from build123d import *

# Parameters (mm, degrees)
SKETCH1_R           = 2.9845
SKETCH1_R_2         = 7.9375
SKETCH1_R_3         = 1.524
SKETCH1_R_4         = 7.250000001
BOSS_EXTRUDE1_DEPTH = 6.35
SKETCH1_3_R         = 7.9375
SKETCH1_3_R_2       = 7.250000001
CUT_EXTRUDE1_DEPTH  = 4.699


with BuildPart() as part:
    # Sketch1 → Boss-Extrude1 (new body)
    # profile 1 of 2: a face of its own
    with BuildSketch(Plane.XY):
        with BuildLine():
            Line((191.225613804, 305.383854225), (112.575613802, 305.383854225))
            ThreePointArc((112.575613802, 305.383854225), (110.330549772, 304.453918255), (109.400613802, 302.208854225))
            Line((109.400613802, 302.208854225), (109.400613802, 218.558854223))
            ThreePointArc((109.400613802, 218.558854223), (110.330549772, 216.313790192), (112.575613802, 215.383854223))
            Line((112.575613802, 215.383854223), (191.225613804, 215.383854223))
            ThreePointArc((191.225613804, 215.383854223), (193.470677834, 216.313790192), (194.400613804, 218.558854223))
            Line((194.400613804, 218.558854223), (194.400613804, 302.208854225))
            ThreePointArc((194.400613804, 302.208854225), (193.470677834, 304.453918255), (191.225613804, 305.383854225))
        make_face()
        with Locations((119.400613802, 245.383854222)):
            Circle(SKETCH1_R, mode=Mode.SUBTRACT)
        with Locations((149.400613802, 245.383854222)):
            Circle(SKETCH1_R, mode=Mode.SUBTRACT)
        with Locations((179.400613802, 225.383854222)):
            Circle(SKETCH1_R_2, mode=Mode.SUBTRACT)
        with Locations((168.605613802, 225.383854222)):
            Circle(SKETCH1_R_3, mode=Mode.SUBTRACT)
        with BuildLine():
            ThreePointArc((119.650613802, 265.633854223), (117.900613802, 263.883854223), (119.650613802, 262.133854222))
            Line((119.650613802, 262.133854222), (128.150613802, 262.133854222))
            ThreePointArc((128.150613802, 262.133854222), (129.900613803, 263.883854223), (128.150613802, 265.633854223))
            Line((128.150613802, 265.633854223), (119.650613802, 265.633854223))
        make_face(mode=Mode.SUBTRACT)
        with BuildLine():
            ThreePointArc((159.150613804, 262.133854222), (160.900613804, 263.883854223), (159.150613804, 265.633854223))
            Line((159.150613804, 265.633854223), (150.650613804, 265.633854223))
            ThreePointArc((150.650613804, 265.633854223), (148.900613803, 263.883854223), (150.650613804, 262.133854222))
            Line((150.650613804, 262.133854222), (159.150613804, 262.133854222))
        make_face(mode=Mode.SUBTRACT)
        with BuildLine():
            ThreePointArc((119.650613802, 296.633854224), (117.900613802, 294.883854224), (119.650613802, 293.133854224))
            Line((119.650613802, 293.133854224), (128.150613802, 293.133854224))
            ThreePointArc((128.150613802, 293.133854224), (129.900613803, 294.883854224), (128.150613802, 296.633854224))
            Line((128.150613802, 296.633854224), (119.650613802, 296.633854224))
        make_face(mode=Mode.SUBTRACT)
        with BuildLine():
            ThreePointArc((159.150613804, 293.133854224), (160.900613804, 294.883854224), (159.150613804, 296.633854224))
            Line((159.150613804, 296.633854224), (150.650613804, 296.633854224))
            ThreePointArc((150.650613804, 296.633854224), (148.900613803, 294.883854224), (150.650613804, 293.133854224))
            Line((150.650613804, 293.133854224), (159.150613804, 293.133854224))
        make_face(mode=Mode.SUBTRACT)
        with BuildLine():
            ThreePointArc((135.400613803, 291.383854224), (123.400613803, 279.383854223), (135.400613803, 267.383854223))
            Line((135.400613803, 267.383854223), (143.400613803, 267.383854223))
            ThreePointArc((143.400613803, 267.383854223), (155.400613803, 279.383854223), (143.400613803, 291.383854224))
            Line((143.400613803, 291.383854224), (135.400613803, 291.383854224))
        make_face(mode=Mode.SUBTRACT)
    # profile 2 of 2: a face of its own
    with BuildSketch(Plane.XY):
        with Locations((179.400613802, 225.383854222)):
            Circle(SKETCH1_R_2)
        with Locations((179.400613802, 225.383854222)):
            Circle(SKETCH1_R_4, mode=Mode.SUBTRACT)
    extrude(amount=BOSS_EXTRUDE1_DEPTH)

    # Sketch1_3 → Cut-Extrude1 (cut)
    with BuildSketch(Plane.XY):
        with Locations((179.400613802, 225.383854222)):
            Circle(SKETCH1_3_R)
        with Locations((179.400613802, 225.383854222)):
            Circle(SKETCH1_3_R_2, mode=Mode.SUBTRACT)
    extrude(amount=CUT_EXTRUDE1_DEPTH, mode=Mode.SUBTRACT)


solid = part.part
Check sheet for the modelled part. Datum: model origin and axes. Units: mm. A direction names the side the tool comes from. Give positions to 0.01 mm unless a question says otherwise; leave off trailing zeros. Order: outer loops, then holes, each group sorted by start corner. A loop starts at its lowest first (then second) coordinate and runs counter-clockwise, first axis right, second up. Notation, with made-up numbers: (74.25, -15.5) - (108.25, -15.5) arc R14 ccw to (108.25, -11.5) - close; hole circle Ø10 at (83, 73). An arc over 180 degrees is marked (long way). Answer as CSV lines item,"result".
1. Section check D-D (z = 2.5). State how many separate pieces and enclosed holes the cut face has, then the cut area to 3 significant figures.
Result sheet:
separate pieces,"1"
enclosed holes,"9"
area,"6,580 mm²"
2. Tool access check on faces 1 (the face through (151, 215.384, 3)), 2 (the face through (186.97, 227.77, 2.32)), 3 (the face through (124, 293.134, 3)). Record the directions out of +Z, -Z, +X, -X, +Y, -Y that give a thin tool (end or side, any length) a straight path to the whole face; none if there is none.
Result sheet:
face 1,"+Z, -Z, +X, -X, -Y"
face 2,"-Z"
face 3,"+Z, -Z"
3. Scan lines: probe 1 along Y at (x, z) = (156.5, 4); probe 2 along Y at (x, z) = (150, 1.5); probe 3 along Y at (x, z) = (142, 0.5). Record each from-to range of solid material in increasing order. Write a range as from..to.
Result sheet:
probe 1,"215.38..262.13, 265.63..293.13, 296.63..305.38"
probe 2,"215.38..242.46, 248.31..262.26, 265.51..269.36, 289.41..293.26, 296.51..305.38"
probe 3,"215.38..267.38, 291.38..305.38"
4. Section check B-B (y = 277.5). Record the boundary of the cut face in (x, z).
Result sheet:
outline,"(109.4, 0) - (123.55, 0) - (123.55, 6.35) - (109.4, 6.35) - close; (155.25, 0) - (194.4, 0) - (194.4, 6.35) - (155.25, 6.35) - close"
5. Go/stop test with a flat-tipped pin: P1, Ø19, axis at x = 179.4, y = 225.38, coming from the -Z side. Record where the tip stops, or that it passes through.
Result sheet:
P1,"z = 0"
6. Mould release check, pull along X, two halves, no side actions. Record for faces 4 (the face through (194.401, 260, 3)), 5 (the face through (110.306, 216.339, 3.131)), 6 (the face through (123.404, 279.648, 3.131)): released by +X, released by -X, zero draft, split by the parting line, or undercut.
Result sheet:
face 4,"released by +X"
face 5,"released by -X"
face 6,"undercut"
7. Section check A-A (x = 158). Record the boundary of the cut face in (y, z).
Result sheet:
outline,"(215.38, 0) - (262.13, 0) - (262.13, 6.35) - (215.38, 6.35) - close; (265.63, 0) - (293.13, 0) - (293.13, 6.35) - (265.63, 6.35) - close; (296.63, 0) - (305.38, 0) - (305.38, 6.35) - (296.63, 6.35) - close"
8. Section check C-C (x = 127). Record the boundary of the cut face in (y, z), then the cut area to 3 significant figures.
Result sheet:
outline,"(215.38, 0) - (262.13, 0) - (262.13, 6.35) - (215.38, 6.35) - close; (265.63, 0) - (270.81, 0) - (270.81, 6.35) - (265.63, 6.35) - close; (287.95, 0) - (293.13, 0) - (293.13, 6.35) - (287.95, 6.35) - close; (296.63, 0) - (305.38, 0) - (305.38, 6.35) - (296.63, 6.35) - close"
area,"418 mm²"
